The listing builds one solid part. Answer for the finished solid, in the listing's coordinates (mm). Give positions to 0.01 mm unless a question says otherwise; leave off trailing zeros. Write each loop counter-clockwise with the first axis right and the second up, starting at its lowest first coordinate (ties: lowest second). Pieces come first, ordered by that corner, then holes. Notation, with made-up numbers: (-25, 25.25) -> (-13, 25.25) arc R26 cw to (-13, 61.25) -> close; hole circle Ø9 at (82, -38). An arc over 180 degrees is marked (long way). Put each result on its own line as item: value. Start each with the question number.
1) A cutting plane is placed at C-C (x = 79). Write down the section's boundary in (y, z) (1 decimal), then the cut area to 3 significant figures.
2) Find the intervals of material crossed by line 1 along Y through (x, z) = (5.25, 0); line 2 along X through (y, z) = (0, -1); line 3 along X through (y, z) = (2, 0), in increasing order. Write a range as from..to.
3) A cutting plane is placed at A-A (y = 0). Write down the section's boundary in (x, z) (1 decimal).
4) Flat-ended cylindrical pins translate along their axes: pin 1 Ø1.5 at (x, y) = (92, 1) entering from -Z; pin 2 Ø5 at (x, z) = (52, -3.5) entering from +Y. Find the tip coordinate at first contact, or state that the pin passes through.
5) A cutting plane is placed at B-B (z = 0). Write down the section's boundary in (x, y) (1 decimal), then the cut area to 3 significant figures.
6) For a pull along Z with two mould halves and no side action, classify faces 1 (the flat face through (0, 1, 2)), 2 (the cylindrical face through (3.502, -0.245, -1.103)), 3 (the cylindrical face through (63.443, -0.209, -4.758)) as released by +Z, released by -Z, zero draft, split by the parting line, or undercut.
from build123d import *

# Parameters (mm, degrees)
SKETCH2_R           = 4.7625
BOSS_EXTRUDE1_DEPTH = 128.651
CHAMFER1_SIZE       = 1.27


# Read off the part's stored shape, not the designer's step: #4-40 Tapped Hole1
with BuildPart() as part:
    # Sketch2 → Boss-Extrude1 (new body)
    with BuildSketch(Plane(origin=(0, 0, 0), x_dir=(0, 0, -1), z_dir=(1, 0, 0))):
        with Locations(Location((0, 0, 0), (0, 0, 180))):
            Circle(SKETCH2_R)
    extrude(amount=BOSS_EXTRUDE1_DEPTH)

    # Chamfer1
    chamfer1_edges = [part.edges().sort_by_distance(p)[0] for p in [
        (0, 0, -4.7625),
        (128.651, 0, -4.7625),
    ]]
    chamfer(chamfer1_edges, length=CHAMFER1_SIZE)

    # Sketch9 → F (0.257) Diameter Hole2 (revolve, cut)
    with BuildSketch(Plane(origin=(9.525, 0, 4.7625), x_dir=(0, -1, 0), z_dir=(1, 0, 0))):
        Polygon((0, 0), (0, 9.525), (3.81, 9.525), (3.2639, 8.9789), (3.2639, 0.5461), (3.81, 0), align=None)
    revolve(axis=Axis((9.525, 0, 11.1125), (0, 0, -1)), mode=Mode.SUBTRACT)

    # #4-40 Tapped Hole1 outline → #4-40 Tapped Hole1 (revolve, cut)
    with BuildSketch(Plane.YX):
        Polygon((1.1303, 0.4572), (1.1303, 6.463087607), (0, 6.463087607), (0, 0), (1.5875, 0), align=None)
    revolve(axis=Axis((0, 0, 0), (1, 0, 0)), mode=Mode.SUBTRACT)


solid = part.part
Reply:
1. outline: circle Ø9.5 at (0, 0)
1. area: 71.3 mm2
2. line 1: y = -4.76..-1.13, 1.13..4.76
2. line 2: x = 12.79..128.65
2. line 3: x = 0..6.95, 12.1..128.65
3. outline: (0, -3.5) -> (1.3, -4.8) -> (5.7, -4.8) -> (6.3, -4.2) -> (6.3, -1.1) -> (0.5, -1.1) -> (0, -1.6) -> close; (0, 1.6) -> (0.5, 1.1) -> (6.3, 1.1) -> (6.3, 4.2) -> (5.7, 4.8) -> (1.3, 4.8) -> (0, 3.5) -> close; (12.8, -4.2) -> (13.3, -4.8) -> (127.4, -4.8) -> (128.7, -3.5) -> (128.7, 3.5) -> (127.4, 4.8) -> (13.3, 4.8) -> (12.8, 4.2) -> close
4. pin 1: stops at z = -4.76
4. pin 2: stops at y = 4.66
5. outline: (0, -3.5) -> (1.3, -4.8) -> (127.4, -4.8) -> (128.7, -3.5) -> (128.7, 3.5) -> (127.4, 4.8) -> (1.3, 4.8) -> (0, 3.5) -> (0, 1.6) -> (0.5, 1.1) -> (6.5, 1.1) arc R3.3 cw (long way) to (6.5, -1.1) -> (0.5, -1.1) -> (0, -1.6) -> close
5. area: 1,170 mm2
6. face 1: zero draft
6. face 2: undercut
6. face 3: split by the parting line
